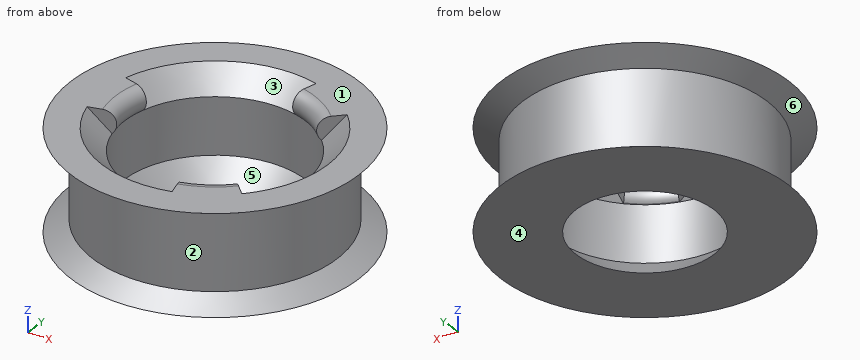
```python
from build123d import *

# Parameters (mm, degrees)
F2_ANGLE_BACK = 15
F2_ANGLE      = 30
F3_COUNT      = 3
F4_R          = 1


with BuildPart() as f1:
    # F0 (on Front) → F1 (revolve)
    with BuildSketch(Plane.XZ):
        Polygon((-7.25, -2.25), (-7.25, 2.25), (-9, 4), (-11.4780508076, 4), (-9.746, 3), (-9.746, -3), (-11.4780508076, -4), (-5.5, -4), align=None)
    revolve(axis=Axis((0, 0, 0), (0, 0, 1)))

    # F0 (on Front) → F2 (revolve)
    with BuildSketch(Plane.XZ, mode=Mode.PRIVATE) as f2_sk:
        Polygon((-9, 4), (-7.25, 2.25), (-5.5, 4), align=None)
    revolve(f2_sk.sketch.rotate(Axis((0, 0, 0), (0, 0, 1)), -F2_ANGLE_BACK), axis=Axis((0, 0, 0), (0, 0, 1)), revolution_arc=F2_ANGLE)

    # F3: F1 ×3 about axis
    f3_axis = Axis((0, 0, 0), (0, 0, 1))


with BuildPart() as f1_1:
    add(f1.part)
    for i in range(1, F3_COUNT):
        add(f1.part.rotate(f3_axis, i * 360 / F3_COUNT))

    # F4
    f4_edges = [f1_1.edges().sort_by_distance(p)[0] for p in [
        (2.75, 4.76314, 4),
        (-5.5, 0, 4),
        (2.75, -4.76314, 4),
    ]]
    fillet(f4_edges, radius=F4_R)


solid = f1_1.part
```
Here's how the part is built. I have some questions about the finished solid (model axes, mm). Face numbers are marked on the shaded views. A direction names the side the tool comes from. Give positions to 0.01 mm unless a question says otherwise; leave off trailing zeros. Loops run counter-clockwise (first coordinate to the right, second up) from the corner with the lowest first, then second, coordinate; pieces in that order, holes last. Notation, with made-up numbers: M 49,72.25 L 92,72.25 A24 ccw 92,88.25 Z; hole C 89.25,-33 d4. An arc over 180 degrees is marked long. Use one line per item in the form item = value. Start each with the question number.
Q1. If we section it at A-A (x = 0): Write out the boundary of the cut face in (y, z), then the cut area to 3 significant figures.
Q2. If we section it at C-C (z = -1): Write out the boundary of the cut face in (x, y), then the cut area to 3 significant figures.
Q3. Thinking about a two-plate mould opening in X: for the marked faces 4, 5 and 6, which applies, +X half, -X half, draft (parallel to the pull), parting line (faces both ways), or undercut?
Q4. If we section it at B-B (y = 0): Write out the boundary of the cut face in (x, z).
Q5. Which directions (+Z, -Z, +X, -X, +Y, -Y) give clear straight access to the entire face, cutting with the end or side of a thin tool? Please do the marked faces 1, 2 and 3.
Q6. Will these pins go through, and if not, where does the flat tip stop? pin 1 Ø4 at (y, z) = (6.5, 2) entering from -X; pin 2 Ø1.5 at (x, z) = (-4, -0.5) entering from -Y; pin 3 Ø1 at (x, z) = (-8, 1.5) entering from +Y.
Q7. I need wall thicknesses on line 1 along X through (y, z) = (0, 0.3); line 2 along X through (y, z) = (4.75, 3.25). Which ranges of each line are inside material? Lowest first, please.
Q8. If we section it at D-D (z = -3.5): Write out the boundary of the cut face in (x, y).
Taken from the geometry:
q1.outline = M -11.48,-4 L -5.5,-4 L -7.25,-2.25 L -7.25,2.25 L -9,4 L -11.48,4 L -9.75,3 L -9.75,-3 Z; M 5.5,-4 L 11.48,-4 L 9.75,-3 L 9.75,3 L 11.48,4 L 9,4 L 7.25,2.25 L 7.25,-2.25 Z
q1.area = 43.4 mm^2
q2.outline = C 0,0 d19.49; hole C 0,0 d14.5
q2.area = 133 mm^2
q3.face_4 = draft
q3.face_5 = undercut
q3.face_6 = parting line
q4.outline = M -11.48,-4 L -5.5,-4 L -7.25,-2.25 L -7.25,2.25 L -7.21,2.29 A1 ccw -7.91,4 L -11.48,4 L -9.75,3 L -9.75,-3 Z; M 5.5,-4 L 11.48,-4 L 9.75,-3 L 9.75,3 L 11.48,4 L 9,4 L 7.25,2.25 L 7.25,-2.25 Z
q5.face_1 = +Z, +X, -X, +Y, -Y
q5.face_2 = none
q5.face_3 = +Z
q6.pin_1 = -9.66
q6.pin_2 = -9.19
q6.pin_3 = 6.22
q7.line_1 = -9.75 to -7.25, 7.25 to 9.75
q7.line_2 = -9 to -6.75, 6.75 to 9
q8.outline = C 0,0 d21.22; hole C 0,0 d12
